For this review, take the finished solid that the model builds, in its own axes (mm). Coordinates: 2 decimals unless noted, no trailing zeros. Write each loop counter-clockwise with the first axis right and the second up, starting at its lowest first coordinate (ties: lowest second). Pieces come first, ordered by that corner, then holes. Notation, with made-up numbers: (-40, -27.75) - (8, -27.75) arc R22 ccw to (8, 0.25) - close; hole circle Ø10 at (17, -36). An arc over 180 degrees is marked (long way). Write each question's results on one line, items separated by ' | '.
from build123d import *

# Parameters (mm, degrees)
BOSS_EXTRUDE1_DEPTH = 1.6


with BuildPart() as part:
    # Sketch1 → Boss-Extrude1 (new body)
    with BuildSketch(Plane(origin=(0, 0, 0), x_dir=(1, 0, 0), z_dir=(0, 1, 0))):
        with BuildLine():
            Line((0, 0), (74.5, 0))
            Line((74.5, 0), (74.5, 22.592093752))
            add(Edge.make_bspline(
                [(74.5, 22.592093752), (65.605442008, 26.625691322), (55.8, 28.490050428)],
                knots=[4.23030835, 4.23030835, 4.23030835, 4.496423735, 4.496423735, 4.496423735], degree=2, weights=[1, 0.991160878, 1]))
            Line((55.8, 28.490050428), (55.8, 16.7))
            Line((55.8, 16.7), (0, 16.7))
            Line((0, 16.7), (0, 0))
        make_face()
    extrude(amount=BOSS_EXTRUDE1_DEPTH)


solid = part.part
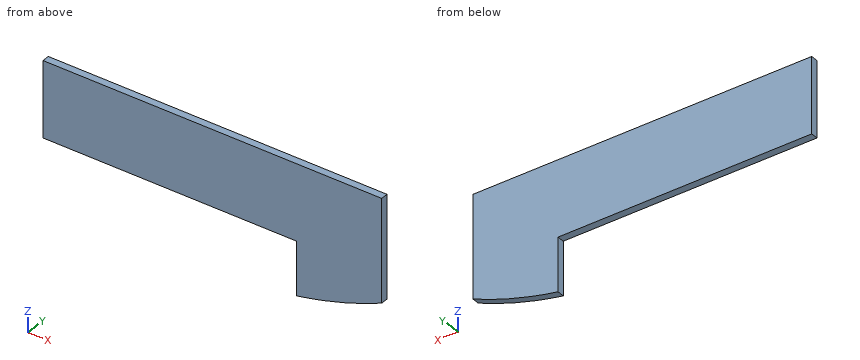
Q1. Take a section at A-A on x = 38.5. State the section outline as (y, z) points.
Results found:
outline: (0, -16.7) - (1.6, -16.7) - (1.6, 0) - (0, 0) - close
Q2. Wall thickness on line 1 along Z through (x, y) = (34, 0.3); line 2 along X through (y, z) = (0.15, -18.5); line 3 along Z through (x, y) = (65, 1.4): over which ranges is each line inside the solid? List them lowest first. Write a range as from..to.
Results found:
line 1: -16.7..0 | line 2: 55.8..74.5 | line 3: -26.2..0
Q3. For pin 1 (5 mm diameter, centred on x = 43.5, z = -19.5, fed in from -Y); pin 2 (0.5 mm diameter, centred on x = 33.5, y = 0.5, fed in from -Z), all flat-tipped, find the tip position at first contact; note any pin that passes through.
Results found:
pin 1: through | pin 2: z = -16.7
Q4. Take a section at B-B on z = -18.25. State the section outline as (x, y) points.
Results found:
outline: (55.8, 0) - (74.5, 0) - (74.5, 1.6) - (55.8, 1.6) - close
